from build123d import *

# Parameters (mm, degrees)
F0_W     = 29
F0_H     = 18
F1_DEPTH = 9
F2_R     = 5
F3_DEPTH = 8
F4_W     = 7
F4_H     = 8
F5_DEPTH = 2
F6_W     = 6
F6_H     = 2
F7_DEPTH = 5
F8_R     = 1.25
F9_DEPTH = 5


with BuildPart() as f1:
    # F0 (on Top) → F1 (new body)
    with BuildSketch(Plane.XY):
        with Locations((14.5, 9)):
            Rectangle(F0_W, F0_H)
    extrude(amount=F1_DEPTH)

    # F2 (on face) → F3 (join)
    with BuildSketch(Plane.XY.offset(9)):
        with Locations((14.5, 9)):
            Circle(F2_R)
    extrude(amount=F3_DEPTH)

    # F4 (on face) → F5 (join)
    with BuildSketch(Plane(origin=(0, 0, 0), x_dir=(1, 0, 0), z_dir=(0, 0, -1))):
        with Locations((21, -12)):
            Rectangle(F4_W, F4_H)
    extrude(amount=F5_DEPTH)

    # F6 (on face) → F7 (join)
    with BuildSketch(Plane(origin=(0, 18, 0), x_dir=(-1, 0, 0), z_dir=(0, 1, 0))):
        with Locations((-13.5, 4)):
            Rectangle(F6_W, F6_H)
    extrude(amount=F7_DEPTH)

    # F8 (on face) → F9 (join)
    with BuildSketch(Plane(origin=(0, 23, 0), x_dir=(-1, 0, 0), z_dir=(0, 1, 0))):
        with Locations((-13.5, 4.25)):
            Circle(F8_R)
    extrude(amount=F9_DEPTH)

    # F12 (on plane+point) → F13 (revolve)
    with BuildSketch(Plane(origin=(0, 0, 4.25), x_dir=(1, 0, 0), z_dir=(0, 0, -1))):
        with BuildLine():
            Line((28.5, -28), (14.75, -28))
            Line((14.75, -28), (13.5, -28))
            Line((13.5, -28), (13.5, -38.8361305416))
            ThreePointArc((13.5, -38.8361305416), (22.7523203186, -35.8437286272), (28.5, -28))
        make_face()
    revolve(axis=Axis((13.5, 35.315773949, 4.25), (0, 1, 0)))


solid = f1.part
For this review, take the finished solid that the model builds, in its own axes (mm). A direction names the side the tool comes from. Round coordinates to 2 decimals unless told otherwise and drop trailing zeros. Loops run counter-clockwise (first coordinate to the right, second up) from the corner with the lowest first, then second, coordinate; pieces in that order, holes last. Notation, with made-up numbers: (78, -5) - (114, -5) arc R20 cw to (114, 10) - close; hole circle Ø4 at (63, 47). An arc over 180 degrees is marked (long way). Put each result on its own line as item: value. Start each with the question number.
1. Insertion check: P1, Ø3.5, axis at x = 20.5, y = 12, coming from the -Z side; P2, Ø1.6, axis at x = 12, z = 3.5, coming from the +Y side; P3, Ø3, axis at x = 3.5, z = 9.5, coming from the -Y side; P4, Ø1.5, axis at x = 14, y = 20.5, coming from the +Z side. Each pin has a flat end and moves straight along its axis. Give the tip position at first contact, or say it passes through.
2. Consider section C-C on z = 1. State the section outline as (x, y) points, plus the area to 3 significant figures.
3. Consider section A-A on y = 9. State the section outline as (x, z) points.
4. For faces 1 (the flat face through (21, 12, -2)), 2 (the flat face through (14, 20, 5)), 3 (the flat face through (21, 16, -1)), 4 (the flat face through (0, 9, 4)), list the 3-axis set-ups (+Z, -Z, +X, -X, +Y, -Y) from which the entire face can be reached by the end or side of a thin tool; tool diameter is ignored.
5. Consider section D-D on x = 26. State the section outline as (y, z) points, plus the area to 3 significant figures.
6. Consider section B-B on x = 16. State the section outline as (y, z) points, plus the area to 3 significant figures.
7. For probe 1 along X at (y, z) = (13.5, 4); probe 2 along Z at (x, y) = (6, 8.5); probe 3 along Y at (x, z) = (7.5, 7.25), list the stretches that pass through material, from the lowest coordinate up. Write a range as [from, to].
Result sheet:
1. P1: z = -2
1. P2: y = 38.81
1. P3: y = 0
1. P4: z = 5
2. outline: (-1.14, 28) - (28.14, 28) arc R15.46 ccw to start; (0, 0) - (29, 0) - (29, 18) - (0, 18) - close
2. area: 747 mm^2
3. outline: (0, 0) - (17.5, 0) - (17.5, -2) - (24.5, -2) - (24.5, 0) - (29, 0) - (29, 9) - (19.5, 9) - (19.5, 17) - (9.5, 17) - (9.5, 9) - (0, 9) - close
4. face 1: -Z, +X, -X, -Y
4. face 2: +Z, +X, -X
4. face 3: -Z, +X, -X
4. face 4: +Z, -Z, -X, -Y
5. outline: (0, 0) - (18, 0) - (18, 9) - (0, 9) - close; (28, -4.04) arc R9.66 ccw to (28, 12.54) - close
5. area: 217 mm^2
6. outline: (0, 0) - (18, 0) - (18, 3) - (23, 3) - (23, 5) - (18, 5) - (18, 9) - (13.77, 9) - (13.77, 17) - (4.23, 17) - (4.23, 9) - (0, 9) - close; (28, -10.54) arc R15.6 ccw to (28, 19.04) - close
6. area: 478 mm^2
7. probe 1: [0, 29]
7. probe 2: [0, 9]
7. probe 3: [0, 18], [28, 37.34]
